Part model, mm, in its own coordinate system. Face numbers are marked on the shaded views. A direction names the side the tool comes from. Coordinates: 2 decimals unless noted, no trailing zeros. Write each loop counter-clockwise with the first axis right and the second up, starting at its lowest first coordinate (ties: lowest second). Pieces come first, ordered by that corner, then holes. Notation, with made-up numbers: M 87.5,11 L 144.5,11 A21 ccw 144.5,28 Z; hole C -19.75,-37.5 d6. An arc over 180 degrees is marked long. Use a Markdown table: item, result. Add a question column.
Q1. Slice it at B-B on z = -2.25. Write the cut outline in (x, y) (3 decimals), then the cut area to 3 significant figures.
Q2. Slice it at C-C on y = 0. Write the cut outline in (x, z), then the cut area to 3 significant figures.
Q3. Tool access for the marked faces 3, 4 and 5: list every direction of +Z, -Z, +X, -X, +Y, -Y with a clear straight run to the whole face (end or side of a thin tool).
Q4. Slice it at A-A on x = -1.5. Write the cut outline in (y, z).
Q5. Pin check, flat tips, straight feed: pin 1 Ø0.5 at (y, z) = (-8, -5.5) entering from +X; pin 2 Ø0.9 at (x, z) = (6, -3.5) entering from +Y (3 decimals); pin 3 Ø0.5 at (x, z) = (5.5, -8.5) entering from -Y (3 decimals). Stop position of each tip, or through.
Q6. Wall check: L1, parallel to Y at x = -1.5, z = -0.7; L2, parallel to Y at x = -1.5, z = -1.65; L3, parallel to Y at x = 3.25, z = -5. Give the ranges that are in metal, low to high. Write a range as from..to.
Q7. Mould opens along Y. For the marked faces 1 and 2 say: released by +Y, released by -Y, zero draft, split by the parting line, or undercut.
Q8. Slice it at D-D on z = -11.75. Write the cut outline in (x, y).
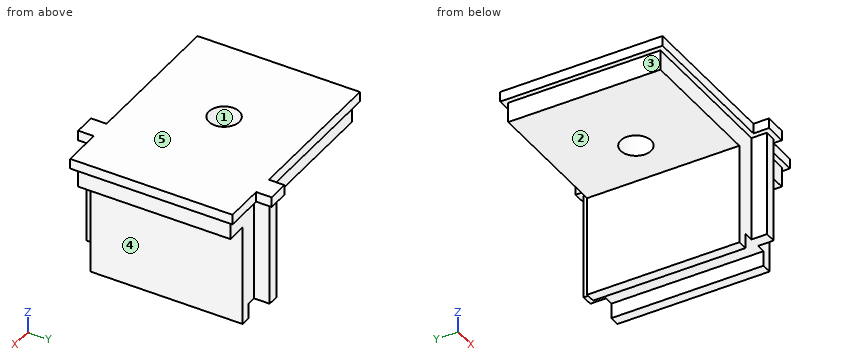
Autodesk Inventor part; units mm, degrees
ref_plane "YZ Plane" through (0, 0, 0) normal (1, 0, 0) x (0, 1, 0)
ref_plane "XZ Plane" through (0, 0, 0) normal (0, 1, 0) x (-1, 0, 0)
ref_plane "XY Plane" through (0, 0, 0) normal (0, 0, 1) x (1, 0, 0)
sketch "Esboço1" plane through (0, 0, 0) normal (0, 0, 1) x (1, 0, 0)
  line L0 (-10, 7.5) -> (10, 7.5)
  line L1 (10, 7.5) -> (10, -7.5)
  line L2 (10, -7.5) -> (-10, -7.5)
  line L3 (-10, -7.5) -> (-10, 7.5)
  line L4 (-10, 7.5) -> (10, -7.5) construction
  line L5 (10, 7.5) -> (-10, -7.5) construction
  circle A0 centre (-1.5, 0) radius 1.5
  point P0 (0, 0)
  dimension "d0" = 20
  dimension "d1" = 15
  dimension "d13" = 3
  dimension "d14" = 1.5
  dimension "d15" = 7.5
extrude "Extrusão1" add sketch "Esboço1" against normal blind 3
sketch "Esboço2" plane through (0, 0, -3) normal (0, 0, -1) x (-1, 0, 0)
  line L0 (10, 7.5) -> (-10, 7.5)
  line L1 (-4, 7.5) -> (-4, -7.5247)
  line L2 (-7, 7.5) -> (-7, -7.5)
  line L3 (-10, -7.5) -> (10, -7.5)
  line L4 (-3, 7.5) -> (-3, -7.5247)
  line L5 (-8, 7.5) -> (-8, -7.5)
  point P0 (0, 0)
  point P1 (0, 0)
  point P2 (-3, -7.5)
  point P3 (-4, -7.5)
  dimension "d6" = 3
  dimension "d7" = 1
  dimension "d8" = 1
  dimension "d16" = 7
extrude "Extrusão2" add sketch "Esboço2" along normal blind 10 contours L4 L3 L1 L0 | L2 L3 L5 L0
sketch "Esboço3" plane through (-10, 7.5, 0) normal (0, 1, 0) x (1, 0, 0)
  point P0 (10, 0)
sketch "Esboço4" plane through (0, 0, -3) normal (0, 0, -1) x (-1, 0, 0)
  line L0 (-7, 7.5) -> (-7, -7.5)
  line L1 (-7, -7.5) -> (-4, -7.5)
  line L2 (-4, -7.5) -> (-4, 7.5)
  line L3 (-4, 7.5) -> (-7, 7.5)
  point P0 (0, 0)
extrude "Extrusão3" add sketch "Esboço4" along normal blind 7
sketch "Sketch5" plane through (0, 0, -10) normal (0, 0, -1) x (-1, 0, 0)
  line L0 (-6.1, 0) -> (-6.1, 9.035)
  line L1 (-6.1, 9.035) -> (-5, 9.035)
  line L2 (-5, 9.035) -> (-5, 0)
  line L3 (-3, 7.5) -> (-8, 7.5)
  line L4 (-7.6007, 9.235) -> (-6.101, 9.235)
  line L5 (-4, 3.5) -> (-4, 7.373)
  line L6 (-7, 7.373) -> (-7, 3.5)
  line L7 (-6.101, -10.265) -> (-7.6007, -10.265)
  line L8 (-11.7517, 0) -> (0.9741, 0)
  line L9 (-6.1, 0) -> (-6.1, -9.035)
  line L10 (-6.1, -9.035) -> (-5, -9.035)
  line L11 (-5, -9.035) -> (-5, 0)
  point P0 (0, 0)
  dimension "d21" = 0.2
  dimension "d22" = 1
  dimension "d23" = 0.9
extrude "Extrusion4" add sketch "Sketch5" against normal blind 10
sketch "Sketch7" plane through (0, 0, 0) normal (0, 0, 1) x (1, 0, 0)
  circle A0 centre (-1.5, 0) radius 1.5
  line L0 (6.1, -7.5) -> (10, -7.5)
  line L1 (10, -7.5) -> (10, 7.5)
  line L2 (10, 7.5) -> (6.1, 7.5)
  line L3 (6.1, 7.5) -> (6.1, 9.035)
  line L4 (6.1, 9.035) -> (5, 9.035)
  line L5 (5, 9.035) -> (5, 7.5)
  line L6 (5, 7.5) -> (-10, 7.5)
  line L7 (-10, 7.5) -> (-10, -7.5)
  line L8 (-10, -7.5) -> (5, -7.5)
  line L9 (5, -7.5) -> (5, -9.035)
  line L10 (5, -9.035) -> (6.1, -9.035)
  line L11 (6.1, -9.035) -> (6.1, -7.5)
  line L12 (10.5, 8) -> (10.5, -8)
  line L13 (10.5, -8) -> (6.6, -8)
  line L14 (6.6, -8) -> (6.6, -9.535)
  line L15 (6.6, -9.535) -> (4.5, -9.535)
  line L16 (4.5, -9.535) -> (4.5, -8)
  line L17 (4.5, -8) -> (-10.5, -8)
  line L18 (-10.5, -8) -> (-10.5, 8)
  line L19 (-10.5, 8) -> (4.5, 8)
  line L20 (4.5, 8) -> (4.5, 9.535)
  line L21 (4.5, 9.535) -> (6.6, 9.535)
  line L22 (6.6, 9.535) -> (6.6, 8)
  line L23 (6.6, 8) -> (10.5, 8)
  circle A1 centre (-1.5, 0) radius 1.5
  point P0 (0, 0)
  dimension "d32" = 0.5
extrude "Extrusion6" add sketch "Sketch7" against normal blind 1 contours L12 L13 L14 L15 L16 L17 L18 L19 L20 L21 L22 L23
sketch "Sketch8" plane through (0, 0, -10) normal (0, 0, -1) x (-1, 0, 0)
  line L0 (-6.1, 7.5) -> (-7, 7.5)
  line L1 (-7, -7.5) -> (-7, 7.5)
  line L2 (-7, -7.5) -> (-6.1, -7.5)
  line L3 (-6.1, -7.5) -> (-6.1, -9.035)
  line L4 (-6.1, -9.035) -> (-5, -9.035)
  line L5 (-5, -9.035) -> (-5, -7.5)
  line L6 (-5, -7.5) -> (-4, -7.5)
  line L7 (-4, 7.5) -> (-4, -7.5)
  line L8 (-4, 7.5) -> (-5, 7.5)
  line L9 (-5, 7.5) -> (-5, 9.035)
  line L10 (-5, 9.035) -> (-6.1, 9.035)
  line L11 (-6.1, 9.035) -> (-6.1, 7.5)
  point P0 (0, 0)
extrude "Extrusion7" add sketch "Sketch8" along normal blind 1.5
properties part number "peca2v2"
Recorded:
| question | item | result |
|---|---|---|
| 1 | outline | M -10,-7.5 L 5,-7.5 L 5,-9.035 L 6.1,-9.035 L 6.1,-7.5 L 10,-7.5 L 10,7.5 L 6.1,7.5 L 6.1,9.035 L 5,9.035 L 5,7.5 L -10,7.5 Z; hole C -1.5,0 d3 |
| 1 | area | 296 mm² |
| 2 | outline | M -10.5,-1 L -10,-1 L -10,-3 L -3,-3 L -3,0 L -10.5,0 Z; M 0,-3 L 3,-3 L 3,-13 L 4,-13 L 4,-11.5 L 7,-11.5 L 7,-13 L 8,-13 L 8,-3 L 10,-3 L 10,-1 L 10.5,-1 L 10.5,0 L 0,0 Z |
| 2 | area | 97.5 mm² |
| 3 | face 3 | -Z, -X, +Y, -Y |
| 3 | face 4 | -Z, +X, +Y, -Y |
| 3 | face 5 | +Z, +X, -X, +Y, -Y |
| 4 | outline | M -8,-1 L -7.5,-1 L -7.5,-3 L -1.5,-3 L -1.5,0 L -8,0 Z; M 1.5,-3 L 7.5,-3 L 7.5,-1 L 8,-1 L 8,0 L 1.5,0 Z |
| 5 | pin 1 | x = 6.1 |
| 5 | pin 2 | y = 9.035 |
| 5 | pin 3 | y = -9.035 |
| 6 | L1 | -8..-1.5, 1.5..8 |
| 6 | L2 | -7.5..-1.5, 1.5..7.5 |
| 6 | L3 | -7.5..7.5 |
| 7 | face 1 | undercut |
| 7 | face 2 | zero draft |
| 8 | outline | M 3,-7.5 L 4,-7.5 L 4,7.5 L 3,7.5 Z; M 7,-7.5 L 8,-7.5 L 8,7.5 L 7,7.5 Z |
